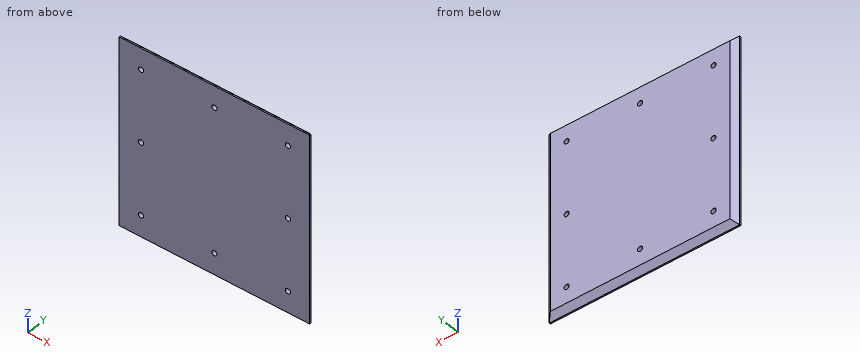
from build123d import *

# Parameters (mm, degrees)
SKETCH1_W           = 177.8
SKETCH1_H           = 177.8
SKETCH1_R           = 2.38125
BOSS_EXTRUDE1_DEPTH = 6.35
CHAMFER1_SIZE       = 5.08


with BuildPart() as part:
    # Sketch1 → Boss-Extrude1 (new body)
    with BuildSketch(Plane(origin=(0, 0, 0), x_dir=(1, 0, 0), z_dir=(0, 1, 0))):
        with Locations((88.9, 88.9)):
            Rectangle(SKETCH1_W, SKETCH1_H)
        with Locations(Location((20.32, 157.48, 0), (0, 0, 270))):
            Circle(SKETCH1_R, mode=Mode.SUBTRACT)
        with Locations(Location((88.9, 157.48, 0), (0, 0, 270))):
            Circle(SKETCH1_R, mode=Mode.SUBTRACT)
        with Locations(Location((157.48, 157.48, 0), (0, 0, 270))):
            Circle(SKETCH1_R, mode=Mode.SUBTRACT)
        with Locations(Location((20.32, 88.9, 0), (0, 0, 270))):
            Circle(SKETCH1_R, mode=Mode.SUBTRACT)
        with Locations(Location((20.32, 20.32, 0), (0, 0, 270))):
            Circle(SKETCH1_R, mode=Mode.SUBTRACT)
        with Locations(Location((88.9, 20.32, 0), (0, 0, 270))):
            Circle(SKETCH1_R, mode=Mode.SUBTRACT)
        with Locations(Location((157.48, 88.9, 0), (0, 0, 270))):
            Circle(SKETCH1_R, mode=Mode.SUBTRACT)
        with Locations(Location((157.48, 20.32, 0), (0, 0, 270))):
            Circle(SKETCH1_R, mode=Mode.SUBTRACT)
    extrude(amount=BOSS_EXTRUDE1_DEPTH)

    # Chamfer1
    chamfer1_edges = [part.edges().sort_by_distance(p)[0] for p in [
        (177.8, 6.35, -88.9),
        (88.9, 6.35, -177.8),
        (0, 6.35, -88.9),
        (88.9, 6.35, 0),
    ]]
    chamfer(chamfer1_edges, length=CHAMFER1_SIZE)


solid = part.part
Geometry: final body of the model. Coordinates: model frame, mm. Give positions to 0.01 mm unless a question says otherwise; leave off trailing zeros. Write each loop counter-clockwise with the first axis right and the second up, starting at its lowest first coordinate (ties: lowest second). Pieces come first, ordered by that corner, then holes.
(1) Cut plane D-D, the plane y = 3.5. Give the number of separate pieces and of enclosed holes in the cut face, then the cut area to 3 significant figures.
(2) Cut plane C-C, the plane z = -88.9. Return loops of the section in (x, y).
(3) Ray query, line 1 (X direction, y = 3.25, z = -88.9); line 2 (X direction, y = 5, z = -20.32); line 3 (Z direction, x = 156, y = 0.5). Return the intervals inside material, ascending.
(4) Cut plane B-B, the plane x = 20.32. Return loops of the section in (y, z).
(5) First-contact query: P1, Ø1, axis at x = 155.5, y = 2.5, coming from the +Z side; P2, Ø4, axis at x = 88.9, z = -157.48, coming from the -Y side. Flat tips, straight axial feed; report the tip coordinate or a pass-through.
(6) Cut plane A-A, the plane z = -20.32. Return loops of the section in (x, y), then the cut area to 3 significant figures.
Values follow:
1. separate pieces: 1
1. enclosed holes: 8
1. area: 29,900 mm2
2. outline: (0, 0) - (17.94, 0) - (17.94, 6.35) - (5.08, 6.35) - (0, 1.27) - close; (22.7, 0) - (155.1, 0) - (155.1, 6.35) - (22.7, 6.35) - close; (159.86, 0) - (177.8, 0) - (177.8, 1.27) - (172.72, 6.35) - (159.86, 6.35) - close
3. line 1: x = 1.98 to 17.94, 22.7 to 155.1, 159.86 to 175.82
3. line 2: x = 3.73 to 17.94, 22.7 to 86.52, 91.28 to 155.1, 159.86 to 174.07
3. line 3: z = -177.8 to -159.35, -155.61 to -90.77, -87.03 to -22.19, -18.45 to 0
4. outline: (0, -177.8) - (1.27, -177.8) - (6.35, -172.72) - (6.35, -159.86) - (0, -159.86) - close; (0, -155.1) - (6.35, -155.1) - (6.35, -91.28) - (0, -91.28) - close; (0, -86.52) - (6.35, -86.52) - (6.35, -22.7) - (0, -22.7) - close; (0, -17.94) - (6.35, -17.94) - (6.35, -5.08) - (1.27, 0) - (0, 0) - close
5. P1: stops at z = -0.73
5. P2: passes through
6. outline: (0, 0) - (17.94, 0) - (17.94, 6.35) - (5.08, 6.35) - (0, 1.27) - close; (22.7, 0) - (86.52, 0) - (86.52, 6.35) - (22.7, 6.35) - close; (91.28, 0) - (155.1, 0) - (155.1, 6.35) - (91.28, 6.35) - close; (159.86, 0) - (177.8, 0) - (177.8, 1.27) - (172.72, 6.35) - (159.86, 6.35) - close
6. area: 1,010 mm2
